Check sheet for the modelled part. Datum: model origin and axes. Units: mm. Face numbers are marked on the shaded views. A direction names the side the tool comes from. Coordinates: 2 decimals unless noted, no trailing zeros. Loops run counter-clockwise (first coordinate to the right, second up) from the corner with the lowest first, then second, coordinate; pieces in that order, holes last. Notation, with made-up numbers: (63, 73.25) -> (102, 73.25) arc R18 ccw to (102, 100.25) -> close; hole circle Ø4 at (12, 85.25). An arc over 180 degrees is marked (long way). Use CSV: the item, a comma, the result in double quotes. Start each with the question number.
1. Sectioned sample at C-C, the plane y = -5. Record the cut outline in (x, z).
2. Sectioned sample at D-D, the plane x = -35.5. Record the cut outline in (y, z).
3. Gauge pin test, flat ends, axial feed: pin 1 (1.1 mm diameter, centred on x = -27.94, z = -6, fed in from +Y); pin 2 (17 mm diameter, centred on x = 21.5, y = -1.5, fed in from +Z); pin 3 (2 mm diameter, centred on x = -27.5, z = -5.5, fed in from +Y); pin 4 (6 mm diameter, centred on x = -25, y = -3.5, fed in from +Z). Record the tip position at first contact, or that the pin passes through.
4. Thickness scan on L1, parallel to Y at x = -23.5, z = -2; L2, parallel to Y at x = 51.5, z = -14.55; L3, parallel to Y at x = -48.5, z = -11. Record the ranges inside material, lowest first.
5. Sectioned sample at A-A, the plane x = -20. Record the cut outline in (y, z), and give its area (3 significant figures).
6. Release check for a two-part mould opening along Y. For the marked faces 1, 2 and 3 record: pulls with the +Y half, pulls with the -Y half, needs draft (parallel to the pull), parting line crosses it, or undercut.
7. Sectioned sample at B-B, the plane z = -11.5. Record the cut outline in (x, y).
8. Set-up check for the marked faces 4 and 5: record each of +Z, -Z, +X, -X, +Y, -Y from which the full face is reachable in a straight line by a thin tool's end or side.
```python
from build123d import *

# Parameters (mm, degrees)
PAD001_DEPTH    = 9.5
SKETCH_R        = 1.6
PAD_DEPTH       = 15
POCKET_DEPTH    = 13
SKETCH003_R     = 10
POCKET001_DEPTH = 15.001
SKETCH004_R     = 0.95
POCKET002_DEPTH = 2
SKETCH005_R     = 3.8
POCKET003_DEPTH = 0.6
SKETCH007_W     = 73.88
SKETCH007_H     = 52.42
POCKET004_DEPTH = 5.5


with BuildPart() as obj1:
    # Sketch006 → Pad001 (new body)
    with BuildSketch(Plane.XY):
        Polygon((-41.25, 27.25), (-29.1, 27.25), (-29.3, 26.05), (-25.7, 26.05), (-25.9, 27.25), (25.9, 27.25), (25.7, 26.05), (29.3, 26.05), (29.1, 27.25), (41.25, 27.25), (41.25, 24.35), (42.85, 24.6), (42.85, 20.4), (41.25, 20.65), (41.25, 1.85), (42.85, 2.1), (42.85, -2.1), (41.25, -1.85), (41.25, -20.65), (42.85, -20.4), (42.85, -24.6), (41.25, -24.35), (41.25, -27.25), (29.35, -27.25), (29.6, -28.85), (25.4, -28.85), (25.65, -27.25), (-25.65, -27.25), (-25.4, -28.85), (-29.6, -28.85), (-29.35, -27.25), (-41.25, -27.25), (-41.25, -24.1), (-40.05, -24.3), (-40.05, -20.7), (-41.25, -20.9), (-41.25, -1.6), (-40.05, -1.8), (-40.05, 1.8), (-41.25, 1.6), (-41.25, 20.9), (-40.05, 20.7), (-40.05, 24.3), (-41.25, 24.1), align=None)
    extrude(amount=-PAD001_DEPTH)


with BuildPart() as body:
    # Sketch → Pad (new body)
    with BuildSketch(Plane.XY):
        with BuildLine():
            Line((-52, 50), (52, 50))
            ThreePointArc((52, 50), (53.06066, 50.43934), (53.5, 51.5))
            Line((53.5, 51.5), (53.5, 55.5))
            ThreePointArc((59, 55.5), (56.25, 58.25), (53.5, 55.5))
            Line((59, 55.5), (59, -35))
            Line((59, -35), (-59, -35))
            Line((-59, 55.5), (-59, -35))
            ThreePointArc((-53.5, 55.5), (-56.25, 58.25), (-59, 55.5))
            Line((-53.5, 51.5), (-53.5, 55.5))
            ThreePointArc((-53.5, 51.5), (-53.06066, 50.43934), (-52, 50))
        make_face()
        with Locations((-56.25, 55.5)):
            Circle(SKETCH_R, mode=Mode.SUBTRACT)
        with Locations((56.25, 55.5)):
            Circle(SKETCH_R, mode=Mode.SUBTRACT)
    extrude(amount=-PAD_DEPTH)

    # Sketch001 (on Face13 of Pad) → Pocket (cut)
    with BuildSketch(Plane.XY):
        with BuildLine():
            Line((-52, 48), (52, 48))
            ThreePointArc((53.5, 46.5), (53.06066, 47.56066), (52, 48))
            Line((53.5, 46.5), (53.5, 36.5))
            ThreePointArc((52, 35), (53.06066, 35.43934), (53.5, 36.5))
            Line((52, 35), (-52, 35))
            ThreePointArc((-53.5, 36.5), (-53.06066, 35.43934), (-52, 35))
            Line((-53.5, 36.5), (-53.5, 46.5))
            ThreePointArc((-52, 48), (-53.06066, 47.56066), (-53.5, 46.5))
        make_face()
    extrude(amount=-POCKET_DEPTH, mode=Mode.SUBTRACT)

    # Sketch003 (on Face4 of Pocket) → Pocket001 (cut, through all)
    with BuildSketch(Plane.XY):
        with Locations((-20, 0)):
            Circle(SKETCH003_R)
        with Locations((20, 0)):
            Circle(SKETCH003_R)
    extrude(amount=-POCKET001_DEPTH, mode=Mode.SUBTRACT)

    # Sketch004 (on Face18 of Pocket001) → Pocket002 (cut)
    with BuildSketch(Plane.XZ.offset(-48)):
        with Locations((-30.48, -6)):
            Circle(SKETCH004_R)
        with Locations((-27.94, -6)):
            Circle(SKETCH004_R)
        with Locations((-25.4, -6)):
            Circle(SKETCH004_R)
        with Locations((-22.86, -6)):
            Circle(SKETCH004_R)
        with Locations((22.86, -6)):
            Circle(SKETCH004_R)
        with Locations((25.4, -6)):
            Circle(SKETCH004_R)
        with Locations((27.94, -6)):
            Circle(SKETCH004_R)
        with Locations((30.48, -6)):
            Circle(SKETCH004_R)
    extrude(amount=-POCKET002_DEPTH, mode=Mode.SUBTRACT)

    # Sketch005 (on Face5 of Pocket002) → Pocket003 (cut)
    with BuildSketch(Plane(origin=(0, 0, -15), x_dir=(1, 0, 0), z_dir=(0, 0, -1))):
        with Locations((-51.5, 27)):
            Circle(SKETCH005_R)
        with Locations((-51.5, -43)):
            Circle(SKETCH005_R)
        with Locations((51.5, -43)):
            Circle(SKETCH005_R)
        with Locations((51.5, 27)):
            Circle(SKETCH005_R)
    extrude(amount=-POCKET003_DEPTH, mode=Mode.SUBTRACT)

    # Boolean: cut obj1
    add(obj1.part, mode=Mode.SUBTRACT)

    # Sketch007 (on Face4 of Boolean) → Pocket004 (cut)
    with BuildSketch(Plane.XY):
        with Locations((-4.31, 1.04)):
            Rectangle(SKETCH007_W, SKETCH007_H)
    extrude(amount=-POCKET004_DEPTH, mode=Mode.SUBTRACT)


solid = body.part
```
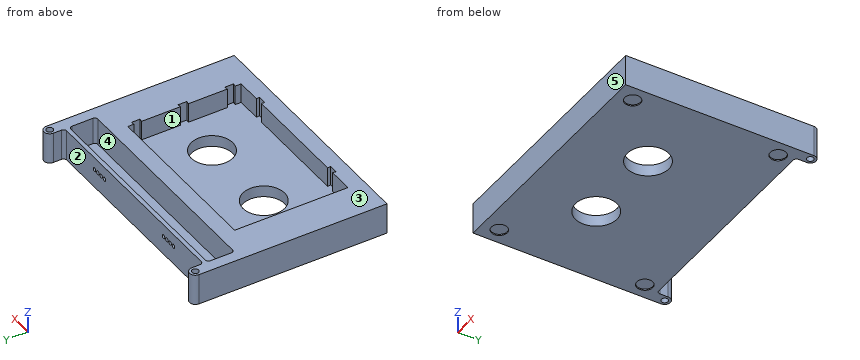
Completed:
1,outline,"(-59, -15) -> (-28.66, -15) -> (-28.66, -9.5) -> (-41.25, -9.5) -> (-41.25, 0) -> (-59, 0) -> close; (-11.34, -15) -> (11.34, -15) -> (11.34, -9.5) -> (-11.34, -9.5) -> close; (28.66, -15) -> (59, -15) -> (59, 0) -> (41.25, 0) -> (41.25, -9.5) -> (28.66, -9.5) -> close"
2,outline,"(-35, -15) -> (50, -15) -> (50, 0) -> (48, 0) -> (48, -13) -> (35, -13) -> (35, 0) -> (27.25, 0) -> (27.25, -9.5) -> (-27.25, -9.5) -> (-27.25, 0) -> (-35, 0) -> close"
3,pin 1,"y = 35"
3,pin 2,"z = -9.5"
3,pin 3,"y = 50"
3,pin 4,"through"
4,L1,"-35 to -27.25, 27.25 to 35, 48 to 50"
4,L2,"-35 to -30.8, -23.2 to 39.2, 46.8 to 50"
4,L3,"-35 to 35, 48 to 50"
5,outline,"(-35, -15) -> (-10, -15) -> (-10, -9.5) -> (-27.25, -9.5) -> (-27.25, 0) -> (-35, 0) -> close; (10, -15) -> (50, -15) -> (50, 0) -> (48, 0) -> (48, -13) -> (35, -13) -> (35, 0) -> (27.25, 0) -> (27.25, -9.5) -> (10, -9.5) -> close"
5,area,"478 mm²"
6,face 1,"undercut"
6,face 2,"pulls with the +Y half"
6,face 3,"needs draft"
7,outline,"(-59, -35) -> (59, -35) -> (59, 55.5) arc R2.75 ccw to (53.5, 55.5) -> (53.5, 51.5) arc R1.5 cw to (52, 50) -> (-52, 50) arc R1.5 cw to (-53.5, 51.5) -> (-53.5, 55.5) arc R2.75 ccw to (-59, 55.5) -> close; hole circle Ø3.2 at (-56.25, 55.5); hole (-53.5, 36.5) arc R1.5 ccw to (-52, 35) -> (52, 35) arc R1.5 ccw to (53.5, 36.5) -> (53.5, 46.5) arc R1.5 ccw to (52, 48) -> (-52, 48) arc R1.5 ccw to (-53.5, 46.5) -> close; hole circle Ø20 at (-20, 0); hole circle Ø20 at (20, 0); hole circle Ø3.2 at (56.25, 55.5)"
8,face 4,"+Z"
8,face 5,"+Z, -Z, +X, -X, -Y"
